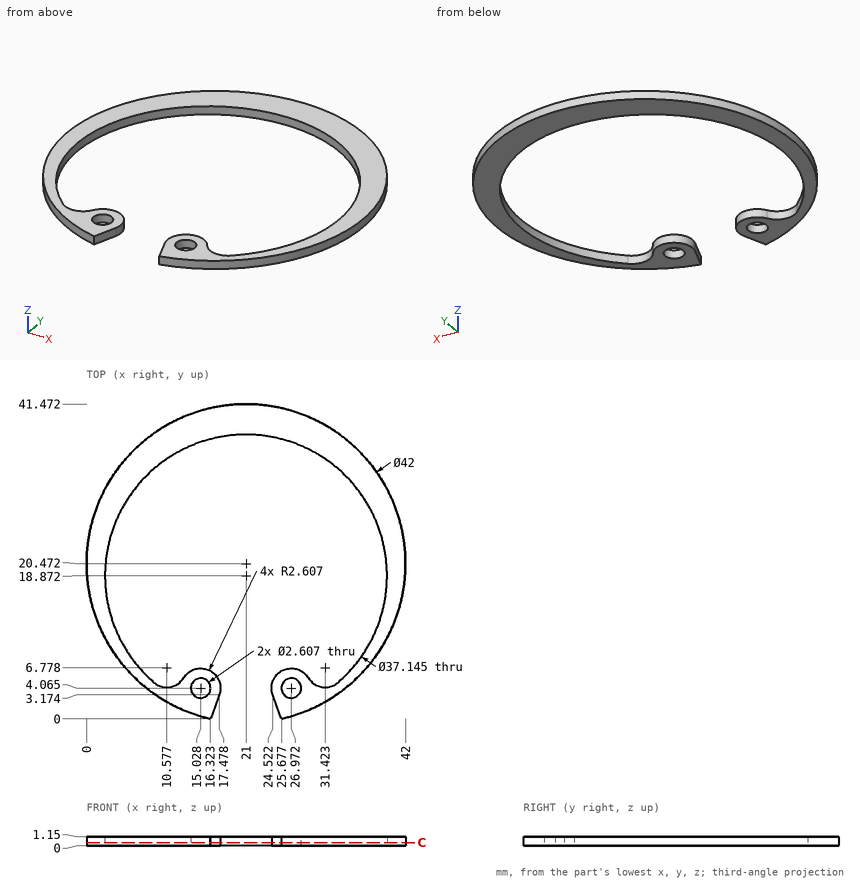
Answer from the drawing. Dimensions are ordinates in mm from the lowest x, y and z of the part. Round coordinates to 2 decimals unless told otherwise and drop trailing zeros. Write each loop counter-clockwise with the first axis right and the second up, starting at its lowest first coordinate (ties: lowest second). Pieces come first, ordered by that corner, then holes. Notation, with made-up numbers: (16, 44) -> (54, 44) arc R10 ccw to (54, 59) -> close; hole circle Ø5 at (32, 21). An arc over 180 degrees is marked (long way). Answer in a Markdown table with one row per item. Add a question column.
1) Given P1, Ø2.5, axis at x = 15.03, y = 4.07, coming from the -Z side; P2, Ø3.5, axis at x = 26.97, y = 4.07, coming from the -Z side, each flat-ended and moving along its own axis, determine where each tip first touches the part or whether it passes through.
2) Consider line 1 (X direction, y = 36, z = 0.3) (1 decimal); line 2 (Y direction, x = 21, z = 0.8) (1 decimal); line 3 (Y direction, x = 11.5, z = 0.25) (1 decimal). Determine where each line is inside the solid, lowest interval first.
3) Find section C-C, the plane z = 0.4. Determine the outline of the cut face in (x, y) (1 decimal).
Findings below:
| question | item | result |
|---|---|---|
| 1 | P1 | through |
| 1 | P2 | z = 0 |
| 2 | line 1 | 6.9 to 13.8, 28.2 to 35.1 |
| 2 | line 2 | 37.4 to 41.5 |
| 2 | line 3 | 1.7 to 4.3, 34.8 to 39.2 |
| 3 | outline | (8.9, 4.8) arc R18.6 cw (long way) to (33.1, 4.8) arc R2.6 cw to (29.2, 5.4) arc R2.6 ccw to (24.5, 3.2) -> (25.7, 0) arc R21 ccw (long way) to (16.3, 0) -> (17.5, 3.2) arc R2.6 ccw to (12.8, 5.4) arc R2.6 cw to start; hole circle Ø2.6 at (15, 4.1); hole circle Ø2.6 at (27, 4.1) |
